Source: CAD feature listing. Evaluate the final solid. Frame: model axes, mm. A direction names the side the tool comes from. Round coordinates to 2 decimals unless told otherwise and drop trailing zeros. Order: outer loops, then holes, each group sorted by start corner. A loop starts at its lowest first (then second) coordinate and runs counter-clockwise, first axis right, second up. Notation, with made-up numbers: (28.25, 28.5) -> (75.25, 28.5) arc R11 ccw to (75.25, 47.5) -> close; hole circle Ø8 at (45, 19). An arc over 180 degrees is marked (long way). Use a Markdown table: item, result. Add a question column.
Autodesk Inventor part; units mm, degrees
ref_plane "YZ Plane" through (0, 0, 0) normal (1, 0, 0) x (0, 1, 0)
ref_plane "XZ Plane" through (0, 0, 0) normal (0, 1, 0) x (-1, 0, 0)
ref_plane "XY Plane" through (0, 0, 0) normal (0, 0, 1) x (1, 0, 0)
sketch "Sketch1" plane through (0, 0, 0) normal (0, 0, 1) x (1, 0, 0)
  line L0 (1.4872, 6.2793) -> (27.4317, 0.1346)
  line L1 (28.584, 0) -> (56, 0)
  line L2 (58, 2) -> (58, 6.4531)
  line L3 (58, 6.4531) -> (66, 6.4531)
  line L4 (66, 6.4531) -> (66, -7)
  line L5 (64, -9) -> (8.701, -9)
  line L6 (7.326, -8.8072) -> (-1.7746, -6.2043)
  arc A0 (1.4872, 6.2793) -> (-1.7746, -6.2043) centre (0, 0) ccw
  arc A1 (27.4317, 0.1346) -> (28.584, 0) centre (28.584, 5) ccw
  arc A2 (7.326, -8.8072) -> (8.701, -9) centre (8.701, -4) ccw
  arc A3 (56, 0) -> (58, 2) centre (56, 2) ccw
  arc A4 (64, -9) -> (66, -7) centre (64, -7) ccw
  point P0 (28, 0)
  point P1 (66, -9)
  point P2 (8, -9)
  point P3 (19, -4)
  dimension "d0" = 66
  dimension "d1" = 8
  dimension "d2" = 9
  dimension "d3" = 20
  dimension "d4" = 28
  dimension "d5" = 5
  dimension "d6" = 2
  dimension "d17" = 45
  dimension "d18" = 4
extrude "Extrusion1" add sketch "Sketch1" along normal mid plane 5
hole "Hole2" at (19, -4, 0) at (0, 0, 0) direction (0, 0, -1) diameter 5.159 end through all both
properties part number "tappy"
1) Section C-C on z = -0.65. Output: boundary loops of the cut face in (x, y), then the cut area to 3 significant figures.
2) Section D-D on y = 1. Output: boundary loops of the cut face in (x, z), then the cut area to 3 significant figures.
3) Reachability of faces 1 (the flat face through (14.28, 3.25, -0.04)), 2 (the cylindrical face through (8.016, -8.953, -0.035)) from +Z, -Z, +X, -X, +Y, -Y: full face, straight path, thin tool, end or side. Return the list, or none.
4) Line query: probe 1 along Y at (x, z) = (19, -0.5); probe 2 along X at (y, z) = (-5.25, -2.05); probe 3 along Y at (x, z) = (0, -0.5). Output: solid intervals per line, ascending. Write a range as from..to.
5) Draft query along X for faces 3 (the flat face through (62, 6.453, 0)), 4 (the cylindrical face through (65.43, -8.4, -0.04)), 5 (the flat face through (42, 0, 0)). Return one class per face: pulls with the +X half, pulls with the -X half, needs draft (parallel to the pull), parting line crosses it, or undercut.
6) Section B-B on y = -4. Output: boundary loops of the cut face in (x, z).
7) First-contact query: pin 1 Ø2 at (y, z) = (5, -1) entering from -X; pin 2 Ø4 at (x, y) = (19, -4) entering from +Z. Flat tips, straight axial feed; report the tip coordinate or a pass-through.
8) Section A-A on x = 0. Output: boundary loops of the cut face in (y, z), then the cut area to 3 significant figures.
Conclusion:
| question | item | result |
|---|---|---|
| 1 | outline | (-1.77, -6.2) -> (7.33, -8.81) arc R5 ccw to (8.7, -9) -> (64, -9) arc R2 ccw to (66, -7) -> (66, 6.45) -> (58, 6.45) -> (58, 2) arc R2 cw to (56, 0) -> (28.58, 0) arc R5 cw to (27.43, 0.13) -> (1.49, 6.28) arc R6.45 ccw to start; hole circle Ø5.16 at (0, 0); hole circle Ø5.16 at (19, -4) |
| 1 | area | 753 mm^2 |
| 2 | outline | (-6.38, -2.5) -> (-2.38, -2.5) -> (-2.38, 2.5) -> (-6.38, 2.5) -> close; (2.38, -2.5) -> (23.78, -2.5) -> (23.78, 2.5) -> (2.38, 2.5) -> close; (57.73, -2.5) -> (66, -2.5) -> (66, 2.5) -> (57.73, 2.5) -> close |
| 2 | area | 168 mm^2 |
| 3 | face 1 | +Z, -Z, +Y |
| 3 | face 2 | +Z, -Z, -X, -Y |
| 4 | probe 1 | y = -9..-6.58, -1.42..2.13 |
| 4 | probe 2 | x = -3.75..16.74, 21.26..66 |
| 4 | probe 3 | y = -6.71..-2.58, 2.58..6.45 |
| 5 | face 3 | needs draft |
| 5 | face 4 | pulls with the +X half |
| 5 | face 5 | undercut |
| 6 | outline | (-5.06, -2.5) -> (16.42, -2.5) -> (16.42, 2.5) -> (-5.06, 2.5) -> close; (21.58, -2.5) -> (66, -2.5) -> (66, 2.5) -> (21.58, 2.5) -> close |
| 7 | pin 1 | stops at x = -5.06 |
| 7 | pin 2 | passes through |
| 8 | outline | (-6.71, -2.5) -> (-2.58, -2.5) -> (-2.58, 2.5) -> (-6.71, 2.5) -> close; (2.58, -2.5) -> (6.45, -2.5) -> (6.45, 2.5) -> (2.58, 2.5) -> close |
| 8 | area | 40.0 mm^2 |
